```python
from build123d import *

# Parameters (mm, degrees)
BOSS_EXTRU_1_DEPTH      = 5
ESQUISSE3_W             = 10
ESQUISSE3_H             = 3
ENL_V_MAT_EXTRU_1_DEPTH = 231.967242256
ENL_V_MAT_EXTRU_2_DEPTH = 231.967242256
ENL_V_MAT_EXTRU_3_DEPTH = 231.967242256
BOSS_EXTRU_2_DEPTH      = 188.5
ESQUISSE6_W             = 3
ESQUISSE6_H             = 4
ENL_V_MAT_EXTRU_4_DEPTH = 221.918340892


with BuildPart() as part:
    # Esquisse1 → Boss.-Extru.1 (new body)
    with BuildSketch(Plane.XY):
        with BuildLine():
            Line((0, 0), (0, -25))
            Line((0, -25), (37.5, -25))
            Line((37.5, -25), (37.5, -95.5))
            Line((37.5, -95.5), (32.5, -95.5))
            Line((32.5, -95.5), (36.487358688, -115.098494092))
            Line((36.487358688, -115.098494092), (88.487358688, -115.098494092))
            Line((88.487358688, -115.098494092), (159.198036807, -44.387815974))
            ThreePointArc((159.198036807, -44.387815974), (187.146342861, -3.044299659), (200.182925478, 45.126663235))
            Line((200.182925478, 45.126663235), (43.682925478, 43.998857528))
            ThreePointArc((43.682925478, 43.998857528), (12.775400091, 31.000392909), (0, 0))
        make_face()
    extrude(amount=BOSS_EXTRU_1_DEPTH)

    # Esquisse3 → Enlèv. mat.-Extru.1 (cut, through all)
    with BuildSketch(Plane.XY.offset(5)):
        with Locations((5, -23.5)):
            Rectangle(ESQUISSE3_W, ESQUISSE3_H)
    extrude(amount=-ENL_V_MAT_EXTRU_1_DEPTH, mode=Mode.SUBTRACT)

    # Esquisse4 → Enlèv. mat.-Extru.2 (cut, through all)
    with BuildSketch(Plane.XY.offset(5)):
        Polygon((88.487358688, -105.098494092), (78.487358688, -105.098494092), (78.487358688, -111.098494092), (68.487358688, -115.098494092), (78.487358688, -115.098494092), (88.487358688, -115.098494092), (98.487358688, -105.098494092), align=None)
    extrude(amount=-ENL_V_MAT_EXTRU_2_DEPTH, mode=Mode.SUBTRACT)

    # Esquisse2 → Enlèv. mat.-Extru.3 (cut, through all)
    with BuildSketch(Plane.XY.offset(5)):
        Polygon((0, 0), (188.5, 0), (209.362190725, -2.460738477), (219.452028236, 63.380017622), (19.477580028, 66.088918501), (-15.632624315, 12.443515375), align=None)
    extrude(amount=-ENL_V_MAT_EXTRU_3_DEPTH, mode=Mode.SUBTRACT)

    # Esquisse5 → Boss.-Extru.2 (add)
    with BuildSketch(Plane.ZY):
        with BuildLine():
            Line((2.5, 0), (5, 0))
            Line((5, 0), (5, 2.5))
            ThreePointArc((5, 2.5), (4.267766953, 0.732233047), (2.5, 0))
        make_face()
        with BuildLine():
            Line((0, 0), (2.5, 0))
            ThreePointArc((2.5, 0), (0.732233047, 0.732233047), (0, 2.5))
            Line((0, 2.5), (0, 0))
        make_face()
    extrude(amount=-BOSS_EXTRU_2_DEPTH)

    # Esquisse6 → Enlèv. mat.-Extru.4 (cut, through all)
    with BuildSketch(Plane(origin=(0, 0, 0), x_dir=(-1, 0, 0), z_dir=(0, 0, -1))):
        with Locations((-53.987358688, -113.098494092)):
            Rectangle(ESQUISSE6_W, ESQUISSE6_H)
    extrude(amount=-ENL_V_MAT_EXTRU_4_DEPTH, mode=Mode.SUBTRACT)


solid = part.part
```
Model file for the job. Use its own axes, mm. A direction names the side the tool comes from. Coordinates: 2 decimals unless noted, no trailing zeros. Order: outer loops, then holes, each group sorted by start corner. A loop starts at its lowest first (then second) coordinate and runs counter-clockwise, first axis right, second up. Notation, with made-up numbers: (34, 19.5) - (79, 19.5) arc R15 ccw to (79, 41.5) - close; hole circle Ø4 at (-7, 13). An arc over 180 degrees is marked (long way). Return JSON: item names as keys, results as strings. Group by question number.
1) Saw through at A-A, the plane x = 84.5. Write the cut outline in (y, z).
2) Saw through at C-C, the plane y = -61. Write the cut outline in (x, z), plus the area to 3 significant figures.
3) Saw through at D-D, the plane x = 24.5. Write the cut outline in (y, z), plus the area to 3 significant figures.
4) Tool access for faces 1 (the flat face through (93, -42, 0)), 2 (the flat face through (52.487, -113, 2)), 3 (the flat face through (78.487, -108, 3)), 4 (the flat face through (35, -95.5, 2)), 5 (the flat face through (5, -22, 3)): list every direction of +Z, -Z, +X, -X, +Y, -Y with a clear straight run to the whole face (end or side of a thin tool).
5) Mould opens along Y. For faces 6 (the flat face through (34.466, -105.162, 2.465)), 7 (the flat face through (37.5, -60, 2)), 8 (the flat face through (93, -44, 5)) say: released by +Y, released by -Y, zero draft, split by the parting line, or undercut.
6) Probe line 1 (Y direction, x = 48, z = 2.8); line 2 (Y direction, x = 13, z = 2.5); line 3 (X direction, y = -100, z = 1). List the from-to ranges inside material, lowest first. Write a range as from..to.
7) Saw through at B-B, the plane z = 0.8. Write the cut outline in (x, y), plus the area to 3 significant figures.
8) Flat gauge pins, fed straight in: P1, Ø1.5, axis at y = -73, z = 1, coming from the -X side; P2, Ø2.5, axis at x = 90, z = 2.5, coming from the -Y side; P3, Ø3, axis at x = 117, z = 2, coming from the +Y side. Where does each tip first touch, or does it go through?
Values found:
{
 "1": {"outline": "(-105.1, 0) - (2.5, 0) arc R2.5 cw to (2.5, 5) - (-105.1, 5) - close"},
 "2": {"outline": "(37.5, 0) - (142.59, 0) - (142.59, 5) - (37.5, 5) - close", "area": "525 mm²"},
 "3": {"outline": "(-25, 0) - (2.5, 0) arc R2.5 cw to (2.5, 5) - (-25, 5) - close", "area": "128 mm²"},
 "4": {"face 1": "-Z, +X, -X, +Y, -Y", "face 2": "+Z, -Z, -Y", "face 3": "+Z, -Z, +X, -Y", "face 4": "+Z, -Z, -X", "face 5": "+Z, -Z, -X, -Y"},
 "5": {"face 6": "released by -Y", "face 7": "undercut", "face 8": "zero draft"},
 "6": {"line 1": "y = -115.1..0.02", "line 2": "y = -25..0", "line 3": "x = 33.42..103.59"},
 "7": {"outline": "(0, -22) - (10, -22) - (10, -25) - (37.5, -25) - (37.5, -95.5) - (32.5, -95.5) - (36.49, -115.1) - (52.49, -115.1) - (52.49, -111.1) - (55.49, -111.1) - (55.49, -115.1) - (68.49, -115.1) - (78.49, -111.1) - (78.49, -105.1) - (98.49, -105.1) - (159.2, -44.39) arc R151.85 ccw to (188.5, 0) - (188.5, 0.67) - (0, 0.67) - close", "area": "13,200 mm²"},
 "8": {"P1": "stops at x = 37.5", "P2": "stops at y = -105.1", "P3": "stops at y = 1"}
}
